Can you work these out from the model? Positions are in its coordinate system, mm. Coordinates: 2 decimals unless noted, no trailing zeros. Order: outer loops, then holes, each group sorted by start corner. A loop starts at its lowest first (then second) coordinate and runs counter-clockwise, first axis right, second up.
```python
from build123d import *

# Parameters (mm, degrees)
SKETCH1_R           = 16
SKETCH1_R_2         = 7.5
BOSS_EXTRUDE1_DEPTH = 4
SKETCH2_R           = 2
CUT_EXTRUDE1_DEPTH  = 42.424630354


with BuildPart() as part:
    # Sketch1 → Boss-Extrude1 (new body)
    # profile 1 of 2: a face of its own
    with BuildSketch(Plane(origin=(0, 0, 0), x_dir=(1, 0, 0), z_dir=(0, 1, 0))):
        Circle(SKETCH1_R)
        with Locations(Location((0, 0, 0), (0, 0, 270))):
            Circle(SKETCH1_R_2, mode=Mode.SUBTRACT)
    # profile 2 of 2: a face of its own
    with BuildSketch(Plane(origin=(0, 0, 0), x_dir=(1, 0, 0), z_dir=(0, 1, 0))):
        with BuildLine():
            Line((38, 16), (0, 16))
            ThreePointArc((0, 16), (11.313708499, 11.313708499), (16, 0))
            ThreePointArc((16, 0), (11.313708499, -11.313708499), (0, -16))
            Line((0, -16), (38, -16))
            Line((38, -16), (38, 16))
        make_face()
    extrude(amount=BOSS_EXTRUDE1_DEPTH)

    # Sketch2 → Cut-Extrude1 (cut, through all)
    with BuildSketch(Plane(origin=(0, 4, 0), x_dir=(1, 0, 0), z_dir=(0, 1, 0))):
        with Locations(Location((30, -8, 0), (0, 0, 270))):
            Circle(SKETCH2_R)
        with Locations(Location((30, 8, 0), (0, 0, 270))):
            Circle(SKETCH2_R)
    extrude(amount=-CUT_EXTRUDE1_DEPTH, mode=Mode.SUBTRACT)


solid = part.part
```
1. Imagine slicing it at D-D on x = -6. Please give me the cut outline in (y, z).
Completed:
outline: (0, -14.83) - (4, -14.83) - (4, -4.5) - (0, -4.5) - close; (0, 4.5) - (4, 4.5) - (4, 14.83) - (0, 14.83) - close
2. Thinking about a two-plate mould opening in X: for faces 1 (the cylindrical face through (0.33, 1.972, -7.493)), 2 (the flat face through (11, 4, 0)), 3 (the cylindrical face through (28, 2, -8)), 4 (the flat face through (38, 2, 0)), which applies, pulls with the +X half, pulls with the -X half, needs draft (parallel to the pull), parting line crosses it, or undercut?
Completed:
face 1: undercut
face 2: needs draft
face 3: undercut
face 4: pulls with the +X half
3. Please list where these lines run through material, in increasing order: probe 1 along X at (y, z) = (2.3, 0); probe 2 along X at (y, z) = (1, 8); probe 3 along Z at (x, y) = (-13, 3.7).
Completed:
probe 1: x = -16 to -7.5, 7.5 to 38
probe 2: x = -13.86 to 28, 32 to 38
probe 3: z = -9.33 to 9.33
4. Imagine slicing it at A-A on x = 30. Please give me the cut outline in (y, z).
Completed:
outline: (0, -16) - (4, -16) - (4, -10) - (0, -10) - close; (0, -6) - (4, -6) - (4, 6) - (0, 6) - close; (0, 10) - (4, 10) - (4, 16) - (0, 16) - close
5. Imagine slicing it at C-C on y = 2.95. Please give me the cut outline in (x, z), then the cut area to 3 significant figures.
Completed:
outline: (0, -16) - (38, -16) - (38, 16) - (0, 16) arc R16 ccw to start; hole circle Ø15 at (0, 0); hole circle Ø4 at (30, -8); hole circle Ø4 at (30, 8)
area: 1,420 mm2
6. Imagine slicing it at B-B on z = 0. Please give me the cut outline in (x, y), then the cut area to 3 significant figures.
Completed:
outline: (-16, 0) - (-7.5, 0) - (-7.5, 4) - (-16, 4) - close; (7.5, 0) - (38, 0) - (38, 4) - (7.5, 4) - close
area: 156 mm2
